Can you work these out from the model? Positions are in its coordinate system, mm. Coordinates: 2 decimals unless noted, no trailing zeros. Write each loop counter-clockwise with the first axis right and the second up, starting at its lowest first coordinate (ties: lowest second). Pieces come first, ordered by that corner, then holes. Notation, with made-up numbers: (30, -2) -> (73, -2) arc R26 ccw to (73, 14) -> close; hole circle Ø2 at (64, 79). An arc over 180 degrees is marked (long way). Use one line per item in the form item = value.
Autodesk Inventor part; units mm, degrees
ref_plane "YZ Plane" through (0, 0, 0) normal (1, 0, 0) x (0, 1, 0)
ref_plane "XZ Plane" through (0, 0, 0) normal (0, 1, 0) x (-1, 0, 0)
ref_plane "XY Plane" through (0, 0, 0) normal (0, 0, 1) x (1, 0, 0)
sketch "Sketch1" plane through (0, 0, 0) normal (0, 1, 0) x (-1, 0, 0)
  line L0 (-1.25, -7.9) -> (1.05, -7.9)
  line L1 (1.05, -7.9) -> (1.05, 7.9)
  line L2 (1.05, 7.9) -> (-1.25, 7.9)
  line L3 (-1.25, 7.9) -> (-1.25, -7.9)
  point P0 (0, 0)
  dimension "d0" = 15.8
  dimension "d7" = 1.05
  dimension "d8" = 1.25
  dimension "d15" = 7.9
extrude "Extrusion1" add sketch "Sketch1" along normal blind 0.6
sketch "Sketch2" plane through (0, 0.6, 0) normal (0, 1, 0) x (1, 0, 0)
  line L0 (0.3, 5.2) -> (-0.3, 5.2)
  line L1 (-0.3, 5.2) -> (-0.3, -5.2)
  line L2 (-0.3, -5.2) -> (0.3, -5.2)
  line L3 (0.3, -5.2) -> (0.3, 5.2)
  line L4 (0.3, 5.2) -> (-0.3, -5.2) construction
  line L5 (-0.3, 5.2) -> (0.3, -5.2) construction
  point P0 (0, 0)
  dimension "d3" = 0.6
  dimension "d4" = 10.4
extrude "Extrusion2" cut sketch "Sketch2" against normal through all
sketch "Sketch3" plane through (0, 0.6, 0) normal (0, 1, 0) x (1, 0, 0)
  line L0 (-1.05, 7.9) -> (-1.05, -7.9)
  line L1 (-1.05, -7.4) -> (-0.55, -7.9)
  line L2 (-1.05, -7.9) -> (1.25, -7.9)
  line L3 (1.25, 7.9) -> (-1.05, 7.9)
  line L4 (-1.05, 7.4) -> (-0.55, 7.9)
  point P0 (0, 0)
  dimension "d9" = 0.5
  dimension "d10" = 0.5
  dimension "d11" = 0.5
  dimension "d12" = 0.5
extrude "Extrusion3" cut sketch "Sketch3" against normal through all
properties part number "insert spacer - v4c"
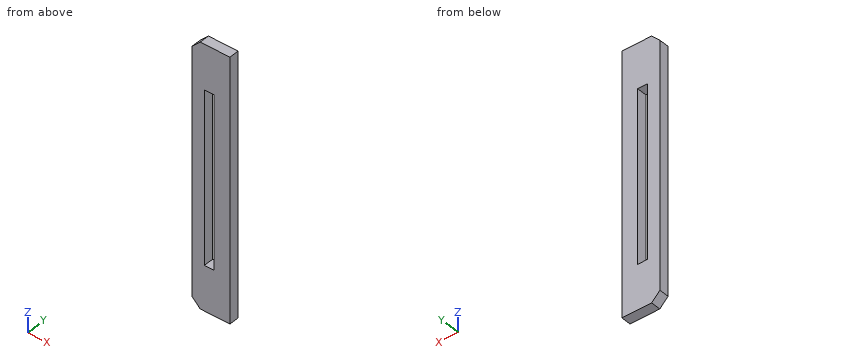
Q1. Suppose I cut it at C-C (y = 0.45). Write out the boundary of the cut face in (x, z).
Return value:
outline = (-1.05, -7.4) -> (-0.55, -7.9) -> (1.25, -7.9) -> (1.25, 7.9) -> (-0.55, 7.9) -> (-1.05, 7.4) -> close; hole (-0.3, -5.2) -> (0.3, -5.2) -> (0.3, 5.2) -> (-0.3, 5.2) -> close
Q2. Suppose I cut it at A-A (x = 0). Write out the boundary of the cut face in (y, z).
Return value:
outline = (0, -7.9) -> (0.6, -7.9) -> (0.6, -5.2) -> (0, -5.2) -> close; (0, 5.2) -> (0.6, 5.2) -> (0.6, 7.9) -> (0, 7.9) -> close
Q3. If I drill on line 1 (X direction, y = 0.4, z = 3); line 2 (Z direction, x = 0, y = 0.25); line 3 (Z direction, x = -0.65, y = 0.4), over which ranges is the centre line in solid material (lowest first)? Write a range as from..to.
Return value:
line_1 = -1.05..-0.3, 0.3..1.25
line_2 = -7.9..-5.2, 5.2..7.9
line_3 = -7.8..7.8
Q4. Suppose I cut it at D-D (x = -0.9). Write out the boundary of the cut face in (y, z).
Return value:
outline = (0, -7.55) -> (0.6, -7.55) -> (0.6, 7.55) -> (0, 7.55) -> close
Q5. Suppose I cut it at B-B (z = 2.75). Write out the boundary of the cut face in (x, y), then the cut area to 3 significant figures.
Return value:
outline = (-1.05, 0) -> (-0.3, 0) -> (-0.3, 0.6) -> (-1.05, 0.6) -> close; (0.3, 0) -> (1.25, 0) -> (1.25, 0.6) -> (0.3, 0.6) -> close
area = 1.02 mm2
